from build123d import *

# Parameters (mm, degrees)
EXTRUDE1_DEPTH     = 10
SKETCH2_R          = 19.5
CUT_EXTRUDE1_DEPTH = 20
SKETCH4_R          = 2.15
CUT_EXTRUDE2_DEPTH = 20


with BuildPart() as part:
    # Sketch1 → Extrude1 (new body)
    with BuildSketch(Plane.XY):
        with BuildLine():
            Line((4, 0), (36, 0))
            ThreePointArc((36, 0), (38.828427125, -1.171572875), (40, -4))
            Line((40, -4), (40, -36))
            ThreePointArc((40, -36), (38.828427125, -38.828427125), (36, -40))
            Line((36, -40), (4, -40))
            ThreePointArc((4, -40), (1.171572875, -38.828427125), (0, -36))
            Line((0, -36), (0, -4))
            ThreePointArc((0, -4), (1.171572875, -1.171572875), (4, 0))
        make_face()
    extrude(amount=EXTRUDE1_DEPTH)

    # Sketch2 → Cut-Extrude1 (cut)
    with BuildSketch(Plane.XY.offset(10)):
        with Locations((20, -20)):
            Circle(SKETCH2_R)
    extrude(amount=-CUT_EXTRUDE1_DEPTH, mode=Mode.SUBTRACT)

    # Sketch4 → Cut-Extrude2 (cut)
    with BuildSketch(Plane.XY.offset(10)):
        with Locations((36, -4)):
            Circle(SKETCH4_R)
        with Locations((4, -4)):
            Circle(SKETCH4_R)
        with Locations((4, -36)):
            Circle(SKETCH4_R)
        with Locations((36, -36)):
            Circle(SKETCH4_R)
    extrude(amount=-CUT_EXTRUDE2_DEPTH, mode=Mode.SUBTRACT)


solid = part.part
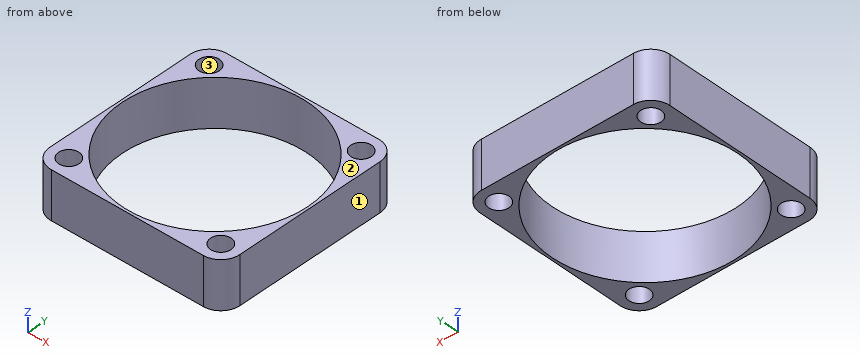
Source: CAD feature listing. Evaluate the final solid. Frame: model axes, mm. Face numbers are marked on the shaded views. Round coordinates to 2 decimals unless told otherwise and drop trailing zeros. Loops run counter-clockwise (first coordinate to the right, second up) from the corner with the lowest first, then second, coordinate; pieces in that order, holes last. Notation, with made-up numbers: M 76,53.5 L 132,53.5 A24 ccw 132,84.5 Z; hole C -19.5,-1.5 d6. An arc over 180 degrees is marked long. Return JSON: item names as keys, results as strings. Group by question number.
1. Material intervals for line 1 along Y through (x, z) = (36, 2.5); line 2 along Y through (x, z) = (19.5, 9.25); line 3 along X through (y, z) = (-2.5, 9.25), sorted ascending. Write a range as from..to.
2. Section query D-D on y = -36.5. Output: boundary loops of the cut face in (x, z), and give its area (3 significant figures).
3. Section query B-B on z = 3.25. Output: boundary loops of the cut face in (x, y), and give its area (3 significant figures).
4. Section query C-C on x = 30. Output: boundary loops of the cut face in (y, z), and give its area (3 significant figures).
5. Section query A-A on y = -20. Output: boundary loops of the cut face in (x, z).
6. Pin query (flat end, axial travel): pin 1 (4 mm diameter, centred on x = 36, y = -4, fed in from +Z). Return the tip coordinate at first contact, or that it passes through.
7. Mould query, pull axis X, two halves, no side actions, for the marked faces 1, 2 and 3. Classes: released by +X, released by -X, zero draft, split by the parting line, or undercut.
Checks:
{
 "1": {"line 1": "y = -40..-38.15, -33.85..-31.15, -8.85..-6.15, -1.85..0", "line 2": "y = -40..-39.49, -0.51..0", "line 3": "x = 0.29..2.46, 5.54..11.4, 28.6..34.46, 37.54..39.71"},
 "2": {"outline": "M 0.03,0 L 1.91,0 L 1.91,10 L 0.03,10 Z; M 6.09,0 L 9.61,0 L 9.61,10 L 6.09,10 Z; M 30.39,0 L 33.91,0 L 33.91,10 L 30.39,10 Z; M 38.09,0 L 39.97,0 L 39.97,10 L 38.09,10 Z", "area": "108 mm²"},
 "3": {"outline": "M 0,-36 A4 ccw 4,-40 L 36,-40 A4 ccw 40,-36 L 40,-4 A4 ccw 36,0 L 4,0 A4 ccw 0,-4 Z; hole C 20,-20 d39; hole C 4,-36 d4.3; hole C 4,-4 d4.3; hole C 36,-36 d4.3; hole C 36,-4 d4.3", "area": "334 mm²"},
 "4": {"outline": "M -40,0 L -36.74,0 L -36.74,10 L -40,10 Z; M -3.26,0 L 0,0 L 0,10 L -3.26,10 Z", "area": "65.2 mm²"},
 "5": {"outline": "M 0,0 L 0.5,0 L 0.5,10 L 0,10 Z; M 39.5,0 L 40,0 L 40,10 L 39.5,10 Z"},
 "6": {"pin 1": "passes through"},
 "7": {"face 1": "released by +X", "face 2": "zero draft", "face 3": "undercut"}
}
